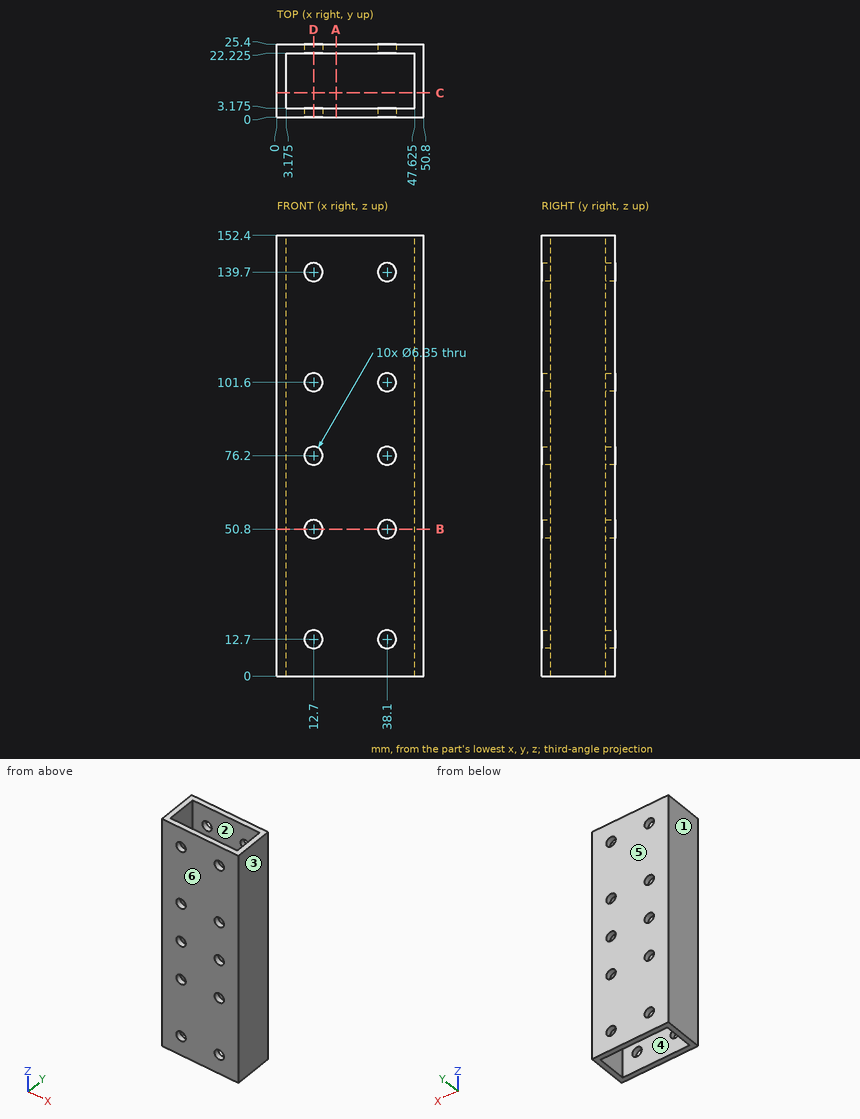
Geometry: see drawing. Coordinates: mm, zero at the bounding-box minimum. A direction names the side the tool comes from. Round coordinates to 2 decimals unless told otherwise and drop trailing zeros. Loops run counter-clockwise (first coordinate to the right, second up) from the corner with the lowest first, then second, coordinate; pieces in that order, holes last. Notation, with made-up numbers: (88.25, 39) -> (122.25, 39) arc R23 cw to (122.25, 63) -> close; hole circle Ø1 at (68, 19). An arc over 180 degrees is marked (long way). Write each question's results on one line, items separated by ' | '.
1. Section B-B (z = 50.8). Return loops of the section in (x, y) (3 decimals).
Geometry results:
outline: (0, 0) -> (9.525, 0) -> (9.525, 3.175) -> (3.175, 3.175) -> (3.175, 22.225) -> (9.525, 22.225) -> (9.525, 25.4) -> (0, 25.4) -> close; (15.875, 0) -> (34.925, 0) -> (34.925, 3.175) -> (15.875, 3.175) -> close; (15.875, 22.225) -> (34.925, 22.225) -> (34.925, 25.4) -> (15.875, 25.4) -> close; (41.275, 0) -> (50.8, 0) -> (50.8, 25.4) -> (41.275, 25.4) -> (41.275, 22.225) -> (47.625, 22.225) -> (47.625, 3.175) -> (41.275, 3.175) -> close
2. Set-up query: the marked faces 1 and 2. Return all of +Z, -Z, +X, -X, +Y, -Y with unobstructed straight access to the full face (end or side cutting, diameter ignored); none if empty.
Geometry results:
face 1: +Z, -Z, -X, +Y, -Y | face 2: +Z, -Z
3. First-contact query: P1, Ø5, axis at x = 12.7, z = 12.7, coming from the +Y side. Flat tip, straight axial feed; report the tip coordinate or a pass-through.
Geometry results:
P1: through
4. Ray query, line 1 (X direction, y = 2.1, z = 139.7) (3 decimals); line 2 (Y direction, x = 13.5, z = 121.5) (3 decimals); line 3 (X direction, y = 8.25, z = 30) (3 decimals). Return the intervals inside material, ascending. Write a range as from..to.
Geometry results:
line 1: 0..9.525, 15.875..34.925, 41.275..50.8 | line 2: 0..3.175, 22.225..25.4 | line 3: 0..3.175, 47.625..50.8
5. Section C-C (y = 8.5). Return loops of the section in (x, z) (3 decimals).
Geometry results:
outline: (0, 0) -> (3.175, 0) -> (3.175, 152.4) -> (0, 152.4) -> close; (47.625, 0) -> (50.8, 0) -> (50.8, 152.4) -> (47.625, 152.4) -> close
6. Section D-D (x = 12.7). State how many separate pieces and enclosed holes the cut face has, and give its area (3 significant figures).
Geometry results:
separate pieces: 12 | enclosed holes: 0 | area: 766 mm2
7. Mould query, pull axis Y, two halves, no side actions, for the marked faces 3, 4, 5 and 6. Classes: +Y half, -Y half, draft (parallel to the pull), parting line (faces both ways), or undercut.
Geometry results:
face 3: draft | face 4: undercut | face 5: +Y half | face 6: -Y half
8. Section A-A (x = 20.5). Return loops of the section in (y, z) (3 decimals), and give its area (3 significant figures).
Geometry results:
outline: (0, 0) -> (3.175, 0) -> (3.175, 152.4) -> (0, 152.4) -> close; (22.225, 0) -> (25.4, 0) -> (25.4, 152.4) -> (22.225, 152.4) -> close | area: 968 mm2
